The listing builds one solid part. Answer for the finished solid, in the listing's coordinates (mm). A direction names the side the tool comes from. Coordinates: 2 decimals unless noted, no trailing zeros. Order: outer loops, then holes, each group sorted by start corner. A loop starts at its lowest first (then second) coordinate and runs counter-clockwise, first axis right, second up.
```python
from build123d import *

# Parameters (mm, degrees)
BOSS_EXTRUDE1_DEPTH = 49.53
FILLET1_R           = 5.08
SKETCH7_R           = 2.2499955
SKETCH7_R_2         = 38.1
CUT_EXTRUDE1_DEPTH  = 26.67
CUT_EXTRUDE2_START  = -7.62
SKETCH8_R           = 3.302
CUT_EXTRUDE2_DEPTH  = 7.62
CUT_EXTRUDE3_DEPTH  = 7.62


with BuildPart() as part:
    # Sketch1 → Boss-Extrude1 (new body, symmetric)
    with BuildSketch(Plane.XY):
        Polygon((0, 0), (0, 171.45), (12.7, 171.45), (12.7, 179.07), (12.7, 199.39), (5.08, 199.39), (5.08, 179.07), (-7.62, 179.07), (-7.62, 171.45), (-7.62, -7.62), (5.08, -7.62), (5.08, -27.94), (12.7, -27.94), (12.7, -7.62), (12.7, 0), align=None)
    extrude(amount=BOSS_EXTRUDE1_DEPTH, both=True)

    # Fillet1
    fillet1_edges = [part.edges().sort_by_distance(p)[0] for p in [
        (5.08, -7.62, 0),
        (-7.62, -7.62, 0),
        (-7.62, 179.07, 0),
        (5.08, 179.07, 0),
        (0, 171.45, 0),
        (0, 0, 0),
    ]]
    fillet(fillet1_edges, radius=FILLET1_R)

    # Sketch7 → Cut-Extrude1 (cut)
    with BuildSketch(Plane(origin=(0, 0, 0), x_dir=(0, 0, -1), z_dir=(1, 0, 0))):
        with Locations((-42.5, 85.725)):
            Circle(SKETCH7_R)
        with Locations((-30.0520382, 115.7770382)):
            Circle(SKETCH7_R)
        with Locations((0, 128.225)):
            Circle(SKETCH7_R)
        with Locations((30.0520382, 115.7770382)):
            Circle(SKETCH7_R)
        with Locations((42.5, 85.725)):
            Circle(SKETCH7_R)
        with Locations((30.0520382, 55.6729618)):
            Circle(SKETCH7_R)
        with Locations((0, 43.225)):
            Circle(SKETCH7_R)
        with Locations((-30.0520382, 55.6729618)):
            Circle(SKETCH7_R)
        with Locations((0, 85.725)):
            Circle(SKETCH7_R_2)
    extrude(amount=-CUT_EXTRUDE1_DEPTH, mode=Mode.SUBTRACT)

    # Sketch8 → Cut-Extrude2 (cut)
    with BuildSketch(Plane.ZY.offset(-5.08).offset(CUT_EXTRUDE2_START)):
        with Locations((-38.1, 191.77)):
            Circle(SKETCH8_R)
        with Locations((0, 191.77)):
            Circle(SKETCH8_R)
        with Locations((38.1, 191.77)):
            Circle(SKETCH8_R)
    cut_extrude2 = extrude(amount=CUT_EXTRUDE2_DEPTH, mode=Mode.SUBTRACT)

    # Mirror1: Cut-Extrude2 across plane
    add(cut_extrude2.mirror(Plane.ZX.offset(85.725)), mode=Mode.SUBTRACT)

    # Sketch14 → Cut-Extrude3 (cut)
    with BuildSketch(Plane.ZY.offset(7.62)):
        with BuildLine():
            Line((12.5, 121.716110013), (12.5, 145.725))
            Line((12.5, 145.725), (-12.5, 145.725))
            Line((-12.5, 145.725), (-12.5, 121.716110013))
            ThreePointArc((-12.5, 121.716110013), (0, 123.825), (12.5, 121.716110013))
        make_face()
    extrude(amount=-CUT_EXTRUDE3_DEPTH, mode=Mode.SUBTRACT)


solid = part.part
```
(1) Consider line 1 (Z direction, x = 9.75, y = 191.77); line 2 (Y direction, x = 10.5, z = 45); line 3 (Y direction, x = -1.5, z = -42.5) (3 decimals). Determine where each line is inside the solid, lowest interval first.
(2) Find section C-C (y = 66). Write down the section's boundary in (x, z), and give its area (3 significant figures).
(3) For faces 4 (the face through (3.552, 180.519, 0.693)), 5 (the face through (9, 171.45, 1)), 6 (the face through (-4, 134, -12.5)), determine the directions among +Z, -Z, +X, -X, +Y, -Y from which every point of the face is accessible in a straight line to the end or side of a thin tool.
(4) Each of these flat-tipped pins is pushed along its axis until it touches: pin 1 Ø8.5 at (x, z) = (-4, 4.5) entering from -Y; pin 2 Ø12 at (y, z) = (-19.5, 7.5) entering from -X; pin 3 Ø7 at (y, z) = (55.67, 30.05) entering from +X; pin 4 Ø4 at (y, z) = (191.77, 38.1) entering from +X. Where does it stop, or does it pass through?
(5) Find section A-A (z = 0). Give the number of separate pieces and of enclosed holes in the cut face, and give its area (3 significant figures).
(6) The mould has two halves that part along Z. Classify faces 1 (the face through (-4, 145.725, 0)), 2 (the face through (8.94, -17.39, 1.52)), 3 (the face through (12.7, 185, 1)): released by +Z, released by -Z, zero draft, split by the parting line, or undercut.
(7) Find section B-B (y = -20.32). Write down the section's boundary in (x, z).
(8) Find section D-D (z = 18.5). Write down the section's boundary in (x, y).
Findings below:
1. line 1: z = -49.53 to -41.4, -34.8 to -3.3, 3.3 to 34.8, 41.4 to 49.53
1. line 2: y = -27.94 to 0, 171.45 to 199.39
1. line 3: y = -7.62 to 83.475, 87.975 to 179.07
2. outline: (-7.62, -49.53) - (0, -49.53) - (0, -32.6) - (-7.62, -32.6) - close; (-7.62, 32.6) - (0, 32.6) - (0, 49.53) - (-7.62, 49.53) - close
2. area: 258 mm2
3. face 4: +Z, -Z, -X, +Y
3. face 5: +Z, -Z, +X
3. face 6: +X, -X
4. pin 1: stops at y = -7.63
4. pin 2: stops at x = 5.08
4. pin 3: stops at x = 0
4. pin 4: passes through
5. separate pieces: 5
5. enclosed holes: 0
5. area: 1,050 mm2
6. face 1: undercut
6. face 2: undercut
6. face 3: zero draft
7. outline: (5.08, -49.53) - (12.7, -49.53) - (12.7, -41.4) - (5.08, -41.4) - close; (5.08, -34.8) - (12.7, -34.8) - (12.7, -3.3) - (5.08, -3.3) - close; (5.08, 3.3) - (12.7, 3.3) - (12.7, 34.8) - (5.08, 34.8) - close; (5.08, 41.4) - (12.7, 41.4) - (12.7, 49.53) - (5.08, 49.53) - close
8. outline: (-7.62, -2.54) arc R5.08 ccw to (-2.54, -7.62) - (0, -7.62) arc R5.08 cw to (5.08, -12.7) - (5.08, -27.94) - (12.7, -27.94) - (12.7, 0) - (5.08, 0) arc R5.08 cw to (0, 5.08) - (0, 52.42) - (-7.62, 52.42) - close; (-7.62, 119.03) - (0, 119.03) - (0, 166.37) arc R5.08 cw to (5.08, 171.45) - (12.7, 171.45) - (12.7, 199.39) - (5.08, 199.39) - (5.08, 184.15) arc R5.08 cw to (0, 179.07) - (-2.54, 179.07) arc R5.08 ccw to (-7.62, 173.99) - close
